Geometry check sheet. Reference: the model listing, model coordinates, mm. A direction names the side the tool comes from. Round coordinates to 2 decimals unless told otherwise and drop trailing zeros. Write each loop counter-clockwise with the first axis right and the second up, starting at its lowest first coordinate (ties: lowest second). Pieces come first, ordered by that corner, then holes.
from build123d import *

# Parameters (mm, degrees)
SKETCH_1_W          = 117
SKETCH_1_H          = 77
EXTRUDE_1_DEPTH     = 17
SKETCH_2_W          = 102
SKETCH_2_H          = 62
CUT_EXTRUDE_1_DEPTH = 15
SKETCH_4_R          = 1.7
CUT_EXTRUDE_2_DEPTH = 73.065942025
SKETCH_5_W          = 7.5
SKETCH_5_H          = 7.5
CUT_EXTRUDE_3_DEPTH = 6
FILLET_2_R          = 1


with BuildPart() as part:
    # ｽｹｯﾁ1 → ﾎﾞｽ - 押し出し1 (new body)
    with BuildSketch(Plane.XY):
        Rectangle(SKETCH_1_W, SKETCH_1_H)
    extrude(amount=EXTRUDE_1_DEPTH)

    # ｽｹｯﾁ2 → ｶｯﾄ - 押し出し1 (cut)
    with BuildSketch(Plane.XY.offset(17)):
        Rectangle(SKETCH_2_W, SKETCH_2_H)
    extrude(amount=-CUT_EXTRUDE_1_DEPTH, mode=Mode.SUBTRACT)

    # ｽｹｯﾁ4 → ｶｯﾄ - 押し出し2 (cut, through all)
    with BuildSketch(Plane(origin=(0, 0, 0), x_dir=(-1, 0, 0), z_dir=(0, 0, -1))):
        with Locations((15, 34.75)):
            Circle(SKETCH_4_R)
        with Locations((15, -34.75)):
            Circle(SKETCH_4_R)
        with Locations((-48.5, -34.75)):
            Circle(SKETCH_4_R)
        with Locations((-48.5, 34.75)):
            Circle(SKETCH_4_R)
    extrude(amount=-CUT_EXTRUDE_2_DEPTH, mode=Mode.SUBTRACT)

    # ｽｹｯﾁ5 → ｶｯﾄ - 押し出し3 (cut)
    with BuildSketch(Plane(origin=(0, 0, 0), x_dir=(-1, 0, 0), z_dir=(0, 0, -1))):
        with Locations((-48.5, -34.75)):
            Rectangle(SKETCH_5_W, SKETCH_5_H)
        with Locations((-48.5, 34.75)):
            Rectangle(SKETCH_5_W, SKETCH_5_H)
        with Locations((15, 34.75)):
            Rectangle(SKETCH_5_W, SKETCH_5_H)
        with Locations((15, -34.75)):
            Rectangle(SKETCH_5_W, SKETCH_5_H)
    extrude(amount=-CUT_EXTRUDE_3_DEPTH, mode=Mode.SUBTRACT)

    # ﾌｨﾚｯﾄ2
    fillet_2_edges = [part.edges().sort_by_distance(p)[0] for p in [
        (44.75, 34.75, 0),
        (52.25, 34.75, 0),
        (48.5, 31, 0),
        (44.75, -34.75, 0),
        (48.5, -31, 0),
        (52.25, -34.75, 0),
        (55.375, 38.5, 0),
        (58.5, 0, 0),
        (-38.625, -38.5, 0),
        (-58.5, 0, 0),
        (16.75, 38.5, 0),
        (-38.625, 38.5, 0),
        (16.75, -38.5, 0),
        (55.375, -38.5, 0),
        (-18.75, -34.75, 0),
        (-15, -31, 0),
        (-11.25, -34.75, 0),
        (-18.75, 34.75, 0),
        (-11.25, 34.75, 0),
        (-15, 31, 0),
    ]]
    fillet(fillet_2_edges, radius=FILLET_2_R)


solid = part.part
1. Scan lines: line 1 along Y through (x, z) = (-15, 9.25); line 2 along Y through (x, z) = (10, 7.75); line 3 along X through (y, z) = (-11, 9). Record each from-to range of solid material in increasing order.
2. Section check A-A (z = 9). Record the cut outline in (x, y), plus the area to 3 significant figures.
3. Section check B-B (x = -15). Record the cut outline in (y, z), plus the area to 3 significant figures.
4. Depth check by flat-ended pin: pin 1 Ø1.5 at (x, y) = (-31, 27) entering from +Z; pin 2 Ø0.5 at (x, z) = (-16.5, 1.5) entering from +Y; pin 3 Ø5.5 at (x, y) = (48.5, -34.75) entering from +Z; pin 4 Ø0.8 at (x, z) = (-16, 1.5) entering from -Y. Enter the tip coordinate at first touch or a pass-through.
5. Release check for a two-part mould opening along X. For faces 1 (the face through (44.75, 35, 3)), 2 (the face through (52.25, 35, 3)), 3 (the face through (58.5, -1, 9)), 4 (the face through (-58.5, -1, 9)) record: +X half, -X half, draft (parallel to the pull), parting line (faces both ways), or undercut.
6. Section check D-D (z = 3.75). Record the cut outline in (x, y), plus the area to 3 significant figures.
7. Access from +Z, -Z, +X, -X, +Y, -Y to the whole of each face (thin tool, end or side, straight path). Record for faces 5 (the face through (-1, -38.5, 9)), 6 (the face through (50.2, 31, 1.8)), 7 (the face through (52.25, -35, 3)), 8 (the face through (-13, 35, 6)).
8. Section check C-C (y = -34.75). Record the cut outline in (x, z).
Results below:
1. line 1: y = -38.5 to -36.45, -33.05 to -31, 31 to 33.05, 36.45 to 38.5
1. line 2: y = -38.5 to -31, 31 to 38.5
1. line 3: x = -58.5 to -51, 51 to 58.5
2. outline: (-58.5, -38.5) - (58.5, -38.5) - (58.5, 38.5) - (-58.5, 38.5) - close; hole (-51, -31) - (51, -31) - (51, 31) - (-51, 31) - close; hole circle Ø3.4 at (-15, -34.75); hole circle Ø3.4 at (-15, 34.75); hole circle Ø3.4 at (48.5, -34.75); hole circle Ø3.4 at (48.5, 34.75)
2. area: 2,650 mm2
3. outline: (-38.5, 6) - (-36.45, 6) - (-36.45, 17) - (-38.5, 17) - close; (-33.05, 6) - (-31, 6) - (-31, 17) - (-33.05, 17) - close; (-31, 1) arc R1 ccw to (-30, 0) - (30, 0) arc R1 ccw to (31, 1) - (31, 2) - (-31, 2) - close; (31, 6) - (33.05, 6) - (33.05, 17) - (31, 17) - close; (36.45, 6) - (38.5, 6) - (38.5, 17) - (36.45, 17) - close
3. area: 214 mm2
4. pin 1: stops at z = 2
4. pin 2: stops at y = 31
4. pin 3: stops at z = 17
4. pin 4: stops at y = -31
5. face 1: undercut
5. face 2: undercut
5. face 3: +X half
5. face 4: -X half
6. outline: (-58.5, -38.5) - (-18.75, -38.5) - (-18.75, -31) - (-51, -31) - (-51, 31) - (-18.75, 31) - (-18.75, 38.5) - (-58.5, 38.5) - close; (-11.25, -38.5) - (44.75, -38.5) - (44.75, -31) - (-11.25, -31) - close; (-11.25, 31) - (44.75, 31) - (44.75, 38.5) - (-11.25, 38.5) - close; (51, -31) - (52.25, -31) - (52.25, -38.5) - (58.5, -38.5) - (58.5, 38.5) - (52.25, 38.5) - (52.25, 31) - (51, 31) - close
6. area: 2,460 mm2
7. face 5: +Z, -Z, +X, -X, -Y
7. face 6: -Z, +Y
7. face 7: -Z, -Y
7. face 8: -Z, +Y, -Y
8. outline: (-58.5, 1) arc R1 ccw to (-57.5, 0) - (-19.75, 0) arc R1 ccw to (-18.75, 1) - (-18.75, 6) - (-16.7, 6) - (-16.7, 17) - (-58.5, 17) - close; (-13.3, 6) - (-11.25, 6) - (-11.25, 1) arc R1 ccw to (-10.25, 0) - (43.75, 0) arc R1 ccw to (44.75, 1) - (44.75, 6) - (46.8, 6) - (46.8, 17) - (-13.3, 17) - close; (50.2, 6) - (52.25, 6) - (52.25, 1) arc R1 ccw to (53.25, 0) - (57.5, 0) arc R1 ccw to (58.5, 1) - (58.5, 17) - (50.2, 17) - close
